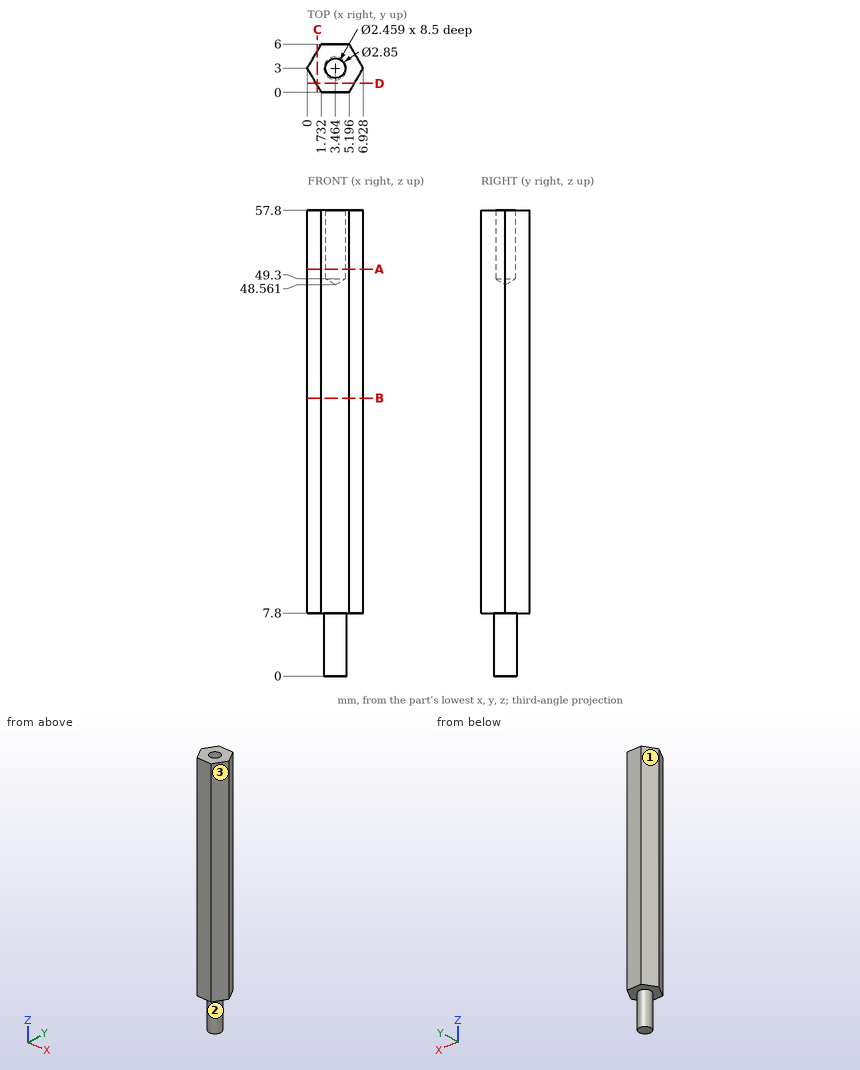
Job drawing, mm, ordinate dimensions from the low corner. One solid piece. Give positions to 0.01 mm unless a question says otherwise; leave off trailing zeros. Write each loop counter-clockwise with the first axis right and the second up, starting at its lowest first coordinate (ties: lowest second). Pieces come first, ordered by that corner, then holes. Notation, with made-up numbers: (11.5, 25.5) - (68.5, 25.5) arc R19 ccw to (68.5, 56.5) - close; hole circle Ø11 at (-12, 60). An arc over 180 degrees is marked (long way). Answer as CSV lines item,"result".
1. Two-plate mould, pull along Y, no slides. Class the marked faces 1, 2 and 3: +Y half, -Y half, draft (parallel to the pull), parting line (faces both ways), or undercut.
Responses:
face 1,"+Y half"
face 2,"parting line"
face 3,"-Y half"
2. Band-saw the part on C-C (x = 1.25). Write the cut outline in (y, z) (1 decimal).
Responses:
outline,"(0.8, 7.8) - (5.2, 7.8) - (5.2, 57.8) - (0.8, 57.8) - close"
3. Band-saw the part on D-D (y = 1.1). Write the cut outline in (x, z).
Responses:
outline,"(1.1, 7.8) - (5.83, 7.8) - (5.83, 57.8) - (1.1, 57.8) - close"
4. Pin check, flat tip, straight feed: pin 1 (1.5 mm diameter, centred on x = 3.46, y = 3, fed in from +Z) (1 decimal). Stop position of the tip, or through.
Responses:
pin 1,"stops at z = 49"
5. Band-saw the part on B-B (z = 34.5). Write the cut outline in (x, y), and give its area (3 significant figures).
Responses:
outline,"(0, 3) - (1.73, 0) - (5.2, 0) - (6.93, 3) - (5.2, 6) - (1.73, 6) - close"
area,"31.2 mm2"
6. Drill centre lines: L1, parallel to X at y = 3, z = 51 (1 decimal); L2, parallel to Y at x = 3.5, z = 54.5; L3, parallel to Z at x = 2.25, y = 4.95. Where is each one in solid material? Low to high. Write a range as [from, to].
Responses:
L1,"x = [0, 2.2], [4.7, 6.9]"
L2,"y = [0, 1.77], [4.23, 6]"
L3,"z = [7.8, 57.8]"
7. Band-saw the part on A-A (z = 50.5). Write the cut outline in (x, y).
Responses:
outline,"(0, 3) - (1.73, 0) - (5.2, 0) - (6.93, 3) - (5.2, 6) - (1.73, 6) - close; hole circle Ø2.46 at (3.46, 3)"
